Autodesk Inventor part; units mm, degrees
ref_plane "YZ Plane" through (0, 0, 0) normal (1, 0, 0) x (0, 1, 0)
ref_plane "XZ Plane" through (0, 0, 0) normal (0, 1, 0) x (-1, 0, 0)
ref_plane "XY Plane" through (0, 0, 0) normal (0, 0, 1) x (1, 0, 0)
sketch "Sketch1" plane through (0, 0, 0) normal (0, 0, 1) x (1, 0, 0)
  circle A0 centre (0, 0) radius 3.5
  circle A1 centre (0, 0) radius 1.5
  circle A2 centre (0, 0) radius 3.05
  dimension "D" = 7
  dimension "M3" = 3
  dimension "d12" = 6.1
extrude "Extrusion1" add sketch "Sketch1" along normal blind 8 contours A0 | A2
sketch "Sketch3" plane through (0, 0, 0) normal (1, 0, 0) x (0, 1, 0)
  line L0 (3.5, 8) -> (3.5, 0)
  line L1 (3.5, 0) -> (1.5, 0)
  line L2 (1.5, 0) -> (1.5, 8)
  line L3 (1.5, 8) -> (3.5, 8)
  line L4 (-3.5, 0) -> (-3.5, 8)
  line L5 (-3.5, 8) -> (-1.5, 8)
  line L6 (-1.5, 8) -> (-1.5, 0)
  line L7 (-1.5, 0) -> (-3.5, 0)
  line L8 (5.6436, 0) -> (3.5, 0)
  line L9 (0, -1.6) -> (0, 9.6)
  line L10 (3.5, 8) -> (5.5, 8)
  line L11 (5.5, 8) -> (7, 0)
  line L12 (7, 0) -> (3.5, 0)
  point P0 (0, 0)
  dimension "d15" = 2
  dimension "d18" = 7
revolve "Revolution2" add sketch "Sketch3" angle 360 about axis through (0, 0, -10) along (0, 0, 1) contours L10 L11 L12 L8 L0
extrude "Extrusion3" cut sketch "Sketch1" along normal up to surface (8 mm away) contours A0 | A2
fillet "Fillet1" radius 0.2 1 edges at (0, -5.5, 8)
extrude "Extrusion4" add sketch "Sketch1" along normal blind 1.5 contours A0 | A2
properties part number "Amortecedor_Borracha" material "Rubber"
Geometry: final body of the model. Coordinates: model frame, mm. A direction names the side the tool comes from. Coordinates: 2 decimals unless noted, no trailing zeros. Loops run counter-clockwise (first coordinate to the right, second up) from the corner with the lowest first, then second, coordinate; pieces in that order, holes last. Notation, with made-up numbers: M 42.5,82.25 L 95.5,82.25 A16 cw 95.5,102.25 Z; hole C 60.5,-6.5 d6. An arc over 180 degrees is marked long. Put each result on its own line as item: value.
(1) Cut plane C-C on z = 4. Return the cut outline in (x, y).
Answer sheet:
outline: C 0,0 d12.5; hole C 0,0 d7
(2) Access query for faces 1 (the face through (3.233, 1.341, 4.704)), 2 (the face through (-2, 0, 0)). Directions: +Z, -Z, +X, -X, +Y, -Y. A direction counts if a zero-diameter tool reaches every point of the face in a straight line with its end or side. Return the directions, or none.
Answer sheet:
face 1: +Z
face 2: -Z, +X, -X, +Y, -Y
(3) First-contact query: pin 1 (3 mm diameter, centred on y = -4.5, z = 2.5, fed in from -X); pin 2 (3.5 mm diameter, centred on x = -1, y = -1.5, fed in from +Z); pin 3 (3.5 mm diameter, centred on x = 0, y = 0, fed in from +Z). Flat tips, straight axial feed; report the tip coordinate or a pass-through.
Answer sheet:
pin 1: stops at x = -5.86
pin 2: stops at z = 8
pin 3: stops at z = 1.5
(4) Cut plane A-A on y = 0. Return the cut outline in (x, z).
Answer sheet:
outline: M -7,0 L -1.5,0 L -1.5,1.5 L -3.5,1.5 L -3.5,8 L -5.33,8 A0.2 ccw -5.53,7.84 Z; M 1.5,0 L 7,0 L 5.53,7.84 A0.2 ccw 5.33,8 L 3.5,8 L 3.5,1.5 L 1.5,1.5 Z
(5) Material intervals for probe 1 along X at (y, z) = (2.75, 4); probe 2 along Z at (x, y) = (1, -2.5); probe 3 along Y at (x, z) = (0, 0.8), sorted ascending.
Answer sheet:
probe 1: x = -5.61 to -2.17, 2.17 to 5.61
probe 2: z = 0 to 1.5
probe 3: y = -6.85 to -1.5, 1.5 to 6.85
(6) Draft query along X for faces 3 (the face through (-5.967, -1.325, 4.734)), 4 (the face through (-1.5, -0.07, 0.74)), 5 (the face through (3.5, 1.1, 8)). Return one class per face: pulls with the +X half, pulls with the -X half, needs draft (parallel to the pull), parting line crosses it, or undercut.
Answer sheet:
face 3: parting line crosses it
face 4: undercut
face 5: needs draft
